Check sheet for the modelled part. Datum: model origin and axes. Units: mm. Give positions to 0.01 mm unless a question says otherwise; leave off trailing zeros. Write each loop counter-clockwise with the first axis right and the second up, starting at its lowest first coordinate (ties: lowest second). Pieces come first, ordered by that corner, then holes. Notation, with made-up numbers: M 41.5,38.25 L 95.5,38.25 A28 cw 95.5,75.25 Z; hole C 86,-8.5 d8. An arc over 180 degrees is marked long. Write item = value, one per line. Start each with the question number.
1) Gauge pin test, flat ends, axial feed: pin 1 (1.2 mm diameter, centred on y = 47.5, z = 0.5, fed in from -X); pin 2 (2.5 mm diameter, centred on x = 14.5, y = 80.5, fed in from +Z). Record the tip position at first contact, or that the pin passes through.
2) Scan lines: L1, parallel to Y at x = 14.5, z = 0.35; L2, parallel to X at y = 44, z = 0.75. Record each from-to range of solid material in increasing order.
3) Sectioned sample at C-C, the plane x = 68. Record the cut outline in (y, z).
4) Sectioned sample at A-A, the plane x = 83.5. Record the cut outline in (y, z).
5) Draft check along Y on faces 1 (the face through (24, 25, 2)), 2 (the face through (47, 48, 1.5)). Enter one of: pulls with the +Y half, pulls with the -Y half, needs draft (parallel to the pull), parting line crosses it, or undercut.
from build123d import *

# Parameters (mm, degrees)
BOSS_EXTRUDE3_DEPTH     = 2
BOSS_EXTRUDE3_2_DEPTH   = 2
BOSS_EXTRUDE3_3_DEPTH   = 2
BOSS_EXTRUDE3_4_DEPTH   = 2
BOSS_EXTRUDE3_5_DEPTH   = 2
BOSS_EXTRUDE3_6_DEPTH   = 2
BOSS_EXTRUDE3_7_DEPTH   = 2
BOSS_EXTRUDE3_8_DEPTH   = 2
BOSS_EXTRUDE3_9_DEPTH   = 2
BOSS_EXTRUDE3_10_DEPTH  = 2
BOSS_EXTRUDE4_OUTLINE_R = 1
BOSS_EXTRUDE4_DEPTH     = 1.5


# Read off the part's stored shape, not the designer's step: Boss-Extrude4
with BuildPart() as part:
    # Model → Boss-Extrude3 (new body)
    with BuildSketch(Plane.XY):
        Polygon((59.84570046, 60.330296093), (59.8457, 60.3111), (59.8457, 60.3027), (59.8613, 60.3027), (59.876264405, 60.302691244), (91.309, 60.2843), (89.13842206, 62.894165109), (89.1181, 62.9186), (89.088037471, 62.928783041), (59.846, 72.8339), align=None)
    extrude(amount=BOSS_EXTRUDE3_DEPTH)



with BuildPart() as body_2:
    # Model → Boss-Extrude3 2 (new body)
    with BuildSketch(Plane.XY):
        Polygon((93.49429954, 76.189703907), (93.4943, 76.2089), (93.4943, 76.2173), (93.4787, 76.2173), (93.463735595, 76.217308756), (62.031, 76.2357), (64.20157794, 73.625834891), (64.2219, 73.6014), (64.251962529, 73.591216959), (93.494, 63.6861), align=None)
    extrude(amount=BOSS_EXTRUDE3_2_DEPTH)


with BuildPart() as body_3:
    # Model → Boss-Extrude3 3 (new body)
    with BuildSketch(Plane.XY):
        Polygon((72.68429954, 91.109703907), (72.6843, 91.1289), (72.6843, 91.1373), (72.6687, 91.1373), (72.653735595, 91.137308756), (41.221, 91.1557), (43.39157794, 88.545834891), (43.4119, 88.5214), (43.441962529, 88.511216959), (72.684, 78.6061), align=None)
    extrude(amount=BOSS_EXTRUDE3_3_DEPTH)


with BuildPart() as body_4:
    # Model → Boss-Extrude3 4 (new body)
    with BuildSketch(Plane.XY):
        Polygon((20.63570046, 80.150296093), (20.6357, 80.1311), (20.6357, 80.1227), (20.6513, 80.1227), (20.666264405, 80.122691244), (52.099, 80.1043), (49.92842206, 82.714165109), (49.9081, 82.7386), (49.878037471, 82.748783041), (20.636, 92.6539), align=None)
    extrude(amount=BOSS_EXTRUDE3_4_DEPTH)


with BuildPart() as body_5:
    # Model → Boss-Extrude3 5 (new body)
    with BuildSketch(Plane.XY):
        Polygon((40.7143, 75.0473), (40.6987, 75.0473), (40.683735595, 75.047308756), (9.251, 75.0657), (11.42157794, 72.455834891), (11.4419, 72.4314), (11.471962529, 72.421216959), (40.714, 62.5161), (40.71429954, 75.019703907), (40.7143, 75.0389), align=None)
    extrude(amount=BOSS_EXTRUDE3_5_DEPTH)


with BuildPart() as body_6:
    # Model → Boss-Extrude3 6 (new body)
    with BuildSketch(Plane.XY):
        Polygon((2.04570046, 60.800296093), (2.0457, 60.7811), (2.0457, 60.7727), (2.0613, 60.7727), (2.076264405, 60.772691244), (33.509, 60.7543), (31.33842206, 63.364165109), (31.3181, 63.3886), (31.288037471, 63.398783041), (2.046, 73.3039), align=None)
    extrude(amount=BOSS_EXTRUDE3_6_DEPTH)


with BuildPart() as body_7:
    # Model → Boss-Extrude3 7 (new body)
    with BuildSketch(Plane.XY):
        Polygon((19.090296093, 36.62429954), (19.0711, 36.6243), (19.0627, 36.6243), (19.0627, 36.6087), (19.062691244, 36.593735595), (19.0443, 5.161), (21.654165109, 7.33157794), (21.6786, 7.3519), (21.688783041, 7.381962529), (31.5939, 36.624), align=None)
    extrude(amount=BOSS_EXTRUDE3_7_DEPTH)


with BuildPart() as body_8:
    # Model → Boss-Extrude3 8 (new body)
    with BuildSketch(Plane.XY):
        Polygon((35.3573, 2.9157), (35.3573, 2.9313), (35.357308756, 2.946264405), (35.3757, 34.379), (32.765834891, 32.20842206), (32.7414, 32.1881), (32.731216959, 32.158037471), (22.8261, 2.916), (35.329703907, 2.91570046), (35.3489, 2.9157), align=None)
    extrude(amount=BOSS_EXTRUDE3_8_DEPTH)


with BuildPart() as body_9:
    # Model → Boss-Extrude3 9 (new body)
    with BuildSketch(Plane.XY):
        Polygon((50.41570046, 4.470296093), (50.4157, 4.4511), (50.4157, 4.4427), (50.4313, 4.4427), (50.446264405, 4.442691244), (81.879, 4.4243), (79.70842206, 7.034165109), (79.6881, 7.0586), (79.658037471, 7.068783041), (50.416, 16.9739), align=None)
    extrude(amount=BOSS_EXTRUDE3_9_DEPTH)


with BuildPart() as body_10:
    # Model → Boss-Extrude3 10 (new body)
    with BuildSketch(Plane.XY):
        Polygon((88.62429954, 31.789703907), (88.6243, 31.8089), (88.6243, 31.8173), (88.6087, 31.8173), (88.593735595, 31.817308756), (57.161, 31.8357), (59.33157794, 29.225834891), (59.3519, 29.2014), (59.381962529, 29.191216959), (88.624, 19.2861), align=None)
    extrude(amount=BOSS_EXTRUDE3_10_DEPTH)


with BuildPart() as part_1:
    add(part.part)

    add(body_2.part)  # Boss-Extrude4 merges body 2

    add(body_3.part)  # Boss-Extrude4 merges body 3

    add(body_4.part)  # Boss-Extrude4 merges body 4

    add(body_5.part)  # Boss-Extrude4 merges body 5

    add(body_6.part)  # Boss-Extrude4 merges body 6

    add(body_7.part)  # Boss-Extrude4 merges body 7

    add(body_8.part)  # Boss-Extrude4 merges body 8

    add(body_9.part)  # Boss-Extrude4 merges body 9

    add(body_10.part)  # Boss-Extrude4 merges body 10
    # Boss-Extrude4 outline → Boss-Extrude4 (add)
    with BuildSketch(Plane.XY):
        Polygon((10, 85), (0, 85), (0, 10), (10, 10), (10, 0), (85, 0), (85, 10), (95, 10), (95, 85), (85, 85), (85, 95), (10, 95), align=None)
        with Locations((14.5, 14.5)):
            Circle(BOSS_EXTRUDE4_OUTLINE_R, mode=Mode.SUBTRACT)
        with BuildLine():
            Line((35.3757, 34.379), (35.357308756, 2.946264405))
            ThreePointArc((35.357308756, 2.946264405), (35.375994273, 2.93215571), (35.379898885, 2.909069831))
            ThreePointArc((35.379898885, 2.909069831), (35.353148575, 2.899873011), (35.329703907, 2.91570046))
            Line((35.329703907, 2.91570046), (22.8261, 2.916))
            Line((22.8261, 2.916), (32.7414, 32.1881))
            Line((32.7414, 32.1881), (35.3757, 34.379))
        make_face(mode=Mode.SUBTRACT)
        with BuildLine():
            Line((19.0443, 5.161), (19.062691244, 36.593735595))
            ThreePointArc((19.062691244, 36.593735595), (19.044005727, 36.60784429), (19.040101115, 36.630930169))
            ThreePointArc((19.040101115, 36.630930169), (19.066851425, 36.640126989), (19.090296093, 36.62429954))
            Line((19.090296093, 36.62429954), (31.5939, 36.624))
            Line((31.5939, 36.624), (21.6786, 7.3519))
            Line((21.6786, 7.3519), (19.0443, 5.161))
        make_face(mode=Mode.SUBTRACT)
        with BuildLine():
            Line((81.879, 4.4243), (50.446264405, 4.442691244))
            ThreePointArc((50.446264405, 4.442691244), (50.43215571, 4.424005727), (50.409069831, 4.420101115))
            ThreePointArc((50.409069831, 4.420101115), (50.399873011, 4.446851425), (50.41570046, 4.470296093))
            Line((50.41570046, 4.470296093), (50.416, 16.9739))
            Line((50.416, 16.9739), (79.6881, 7.0586))
            Line((79.6881, 7.0586), (81.879, 4.4243))
        make_face(mode=Mode.SUBTRACT)
        with Locations((80.5, 14.5)):
            Circle(BOSS_EXTRUDE4_OUTLINE_R, mode=Mode.SUBTRACT)
        with BuildLine():
            Line((57.161, 31.8357), (88.593735595, 31.817308756))
            ThreePointArc((88.593735595, 31.817308756), (88.60784429, 31.835994273), (88.630930169, 31.839898885))
            ThreePointArc((88.630930169, 31.839898885), (88.640126989, 31.813148575), (88.62429954, 31.789703907))
            Line((88.62429954, 31.789703907), (88.624, 19.2861))
            Line((88.624, 19.2861), (59.3519, 29.2014))
            Line((59.3519, 29.2014), (57.161, 31.8357))
        make_face(mode=Mode.SUBTRACT)
        with BuildLine():
            Line((10, 42), (10, 53))
            ThreePointArc((10, 53), (11.5, 54.5), (13, 53))
            Line((13, 53), (13, 42))
            ThreePointArc((13, 42), (11.5, 40.5), (10, 42))
        make_face(mode=Mode.SUBTRACT)
        with BuildLine():
            Line((20, 42), (20, 53))
            ThreePointArc((20, 53), (21.5, 54.5), (23, 53))
            Line((23, 53), (23, 42))
            ThreePointArc((23, 42), (21.5, 40.5), (20, 42))
        make_face(mode=Mode.SUBTRACT)
        with BuildLine():
            Line((33.509, 60.7543), (2.076264405, 60.772691244))
            ThreePointArc((2.076264405, 60.772691244), (2.06215571, 60.754005727), (2.039069831, 60.750101115))
            ThreePointArc((2.039069831, 60.750101115), (2.029873011, 60.776851425), (2.04570046, 60.800296093))
            Line((2.04570046, 60.800296093), (2.046, 73.3039))
            Line((2.046, 73.3039), (31.3181, 63.3886))
            Line((31.3181, 63.3886), (33.509, 60.7543))
        make_face(mode=Mode.SUBTRACT)
        with BuildLine():
            Line((9.251, 75.0657), (40.683735595, 75.047308756))
            ThreePointArc((40.683735595, 75.047308756), (40.69784429, 75.065994273), (40.720930169, 75.069898885))
            ThreePointArc((40.720930169, 75.069898885), (40.730126989, 75.043148575), (40.71429954, 75.019703907))
            Line((40.71429954, 75.019703907), (40.714, 62.5161))
            Line((40.714, 62.5161), (11.4419, 72.4314))
            Line((11.4419, 72.4314), (9.251, 75.0657))
        make_face(mode=Mode.SUBTRACT)
        with Locations((14.5, 80.5)):
            Circle(BOSS_EXTRUDE4_OUTLINE_R, mode=Mode.SUBTRACT)
        with BuildLine():
            Line((52.099, 80.1043), (20.666264405, 80.122691244))
            ThreePointArc((20.666264405, 80.122691244), (20.65215571, 80.104005727), (20.629069831, 80.100101115))
            ThreePointArc((20.629069831, 80.100101115), (20.619873011, 80.126851425), (20.63570046, 80.150296093))
            Line((20.63570046, 80.150296093), (20.636, 92.6539))
            Line((20.636, 92.6539), (49.9081, 82.7386))
            Line((49.9081, 82.7386), (52.099, 80.1043))
        make_face(mode=Mode.SUBTRACT)
        with BuildLine():
            Line((72, 42), (72, 53))
            ThreePointArc((72, 53), (73.5, 54.5), (75, 53))
            Line((75, 53), (75, 42))
            ThreePointArc((75, 42), (73.5, 40.5), (72, 42))
        make_face(mode=Mode.SUBTRACT)
        with BuildLine():
            Line((82, 42), (82, 53))
            ThreePointArc((82, 53), (83.5, 54.5), (85, 53))
            Line((85, 53), (85, 42))
            ThreePointArc((85, 42), (83.5, 40.5), (82, 42))
        make_face(mode=Mode.SUBTRACT)
        with BuildLine():
            Line((91.309, 60.2843), (59.876264405, 60.302691244))
            ThreePointArc((59.876264405, 60.302691244), (59.86215571, 60.284005727), (59.839069831, 60.280101115))
            ThreePointArc((59.839069831, 60.280101115), (59.829873011, 60.306851425), (59.84570046, 60.330296093))
            Line((59.84570046, 60.330296093), (59.846, 72.8339))
            Line((59.846, 72.8339), (89.1181, 62.9186))
            Line((89.1181, 62.9186), (91.309, 60.2843))
        make_face(mode=Mode.SUBTRACT)
        with BuildLine():
            Line((62.031, 76.2357), (93.463735595, 76.217308756))
            ThreePointArc((93.463735595, 76.217308756), (93.47784429, 76.235994273), (93.500930169, 76.239898885))
            ThreePointArc((93.500930169, 76.239898885), (93.510126989, 76.213148575), (93.49429954, 76.189703907))
            Line((93.49429954, 76.189703907), (93.494, 63.6861))
            Line((93.494, 63.6861), (64.2219, 73.6014))
            Line((64.2219, 73.6014), (62.031, 76.2357))
        make_face(mode=Mode.SUBTRACT)
        with BuildLine():
            Line((41.221, 91.1557), (72.653735595, 91.137308756))
            ThreePointArc((72.653735595, 91.137308756), (72.66784429, 91.155994273), (72.690930169, 91.159898885))
            ThreePointArc((72.690930169, 91.159898885), (72.700126989, 91.133148575), (72.68429954, 91.109703907))
            Line((72.68429954, 91.109703907), (72.684, 78.6061))
            Line((72.684, 78.6061), (43.4119, 88.5214))
            Line((43.4119, 88.5214), (41.221, 91.1557))
        make_face(mode=Mode.SUBTRACT)
        with Locations((80.5, 80.5)):
            Circle(BOSS_EXTRUDE4_OUTLINE_R, mode=Mode.SUBTRACT)
    extrude(amount=BOSS_EXTRUDE4_DEPTH)


solid = part_1.part
Data:
q1.pin_1 = 0
q1.pin_2 = 1.5
q2.L1 = 0 to 13.5, 15.5 to 79.5, 81.5 to 95
q2.L2 = 0 to 10, 13 to 20, 23 to 72, 75 to 82, 85 to 95
q3.outline = M 0,0 L 95,0 L 95,1.5 L 91.14,1.5 L 91.14,2 L 80.19,2 L 80.19,1.5 L 76.23,1.5 L 76.23,2 L 72.32,2 L 72.32,1.5 L 70.07,1.5 L 70.07,2 L 60.3,2 L 60.3,1.5 L 31.83,1.5 L 31.83,2 L 26.27,2 L 26.27,1.5 L 11.02,1.5 L 11.02,2 L 4.43,2 L 4.43,1.5 L 0,1.5 Z
q4.outline = M 0,0 L 40.5,0 L 40.5,1.5 L 31.82,1.5 L 31.82,2 L 21.02,2 L 21.02,1.5 L 0,1.5 Z; M 54.5,0 L 95,0 L 95,1.5 L 76.22,1.5 L 76.22,2 L 67.07,2 L 67.07,1.5 L 64.82,1.5 L 64.82,2 L 60.29,2 L 60.29,1.5 L 54.5,1.5 Z
q5.face_1 = needs draft
q5.face_2 = undercut
